CAD build for the part. Positions are in the model's coordinates, mm. Face numbers are marked on the shaded views. A direction names the side the tool comes from. Round coordinates to 2 decimals unless told otherwise and drop trailing zeros. Loops run counter-clockwise (first coordinate to the right, second up) from the corner with the lowest first, then second, coordinate; pieces in that order, holes last. Notation, with made-up numbers: (83.25, 23) -> (108.25, 23) arc R34 ccw to (108.25, 61) -> close; hole circle Ø5 at (6, 24.5). An arc over 180 degrees is marked (long way). Answer as CSV lines item,"result".
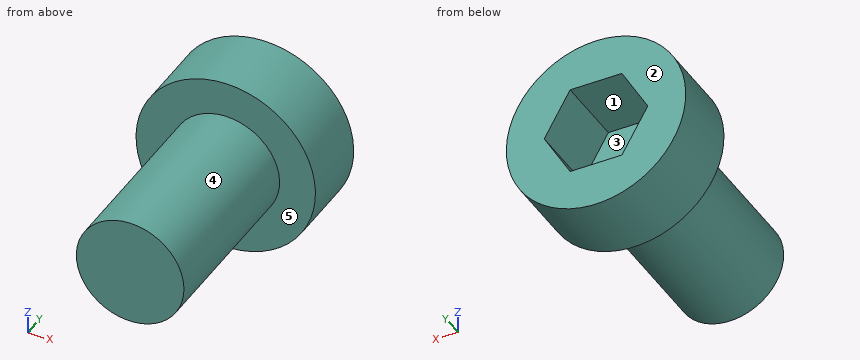
```python
from build123d import *

# Parameters (mm, degrees)
SKETCH1_R      = 3
EXTRUDE1_DEPTH = 10
SKETCH2_R      = 5
EXTRUDE2_DEPTH = 4


with BuildPart() as part:
    # Sketch1 → Extrude1 (new body)
    with BuildSketch(Plane(origin=(0, 0, 0), x_dir=(1, 0, 0), z_dir=(0, 1, 0))):
        with Locations(Location((0, 0, 0), (0, 0, 270))):
            Circle(SKETCH1_R)
    extrude(amount=-EXTRUDE1_DEPTH)

    # Sketch2 → Extrude2 (add)
    with BuildSketch(Plane(origin=(0, 0, 0), x_dir=(1, 0, 0), z_dir=(0, 1, 0))):
        with Locations(Location((0, 0, 0), (0, 0, 270))):
            Circle(SKETCH2_R)
        Polygon((2.886751346, 0), (1.443375673, 2.5), (-1.443375673, 2.5), (-2.886751346, 0), (-1.443375673, -2.5), (1.443375673, -2.5), align=None, mode=Mode.SUBTRACT)
    extrude(amount=EXTRUDE2_DEPTH)


solid = part.part
```
Q1. Slice it at D-D, the plane y = -4.5. Give the cut face in (x, z).
Results:
outline,"circle Ø6 at (0, 0)"
Q2. Slice it at B-B, the plane x = 0. Give the cut face in (y, z).
Results:
outline,"(-10, -3) -> (0, -3) -> (0, -5) -> (4, -5) -> (4, -2.5) -> (0, -2.5) -> (0, 2.5) -> (4, 2.5) -> (4, 5) -> (0, 5) -> (0, 3) -> (-10, 3) -> close"
Q3. Probe L1, parallel to Y at x = 0.75, z = 0; L2, parallel to Y at x = 2.75, z = -2; L3, parallel to Z at x = 2.75, y = 3.25. List the from-to ranges inside material, lowest first. Write a range as [from, to].
Results:
L1,"[-10, 0]"
L2,"[0, 4]"
L3,"[-4.18, -0.24], [0.24, 4.18]"
Q4. Two-plate mould, pull along X, no slides. Class the marked faces 3, 4 and 5: pulls with the +X half, pulls with the -X half, needs draft (parallel to the pull), parting line crosses it, or undercut.
Results:
face 3,"undercut"
face 4,"parting line crosses it"
face 5,"needs draft"
Q5. Drop flat-ended pins along their axis: pin 1 Ø4 at (x, y) = (1.5, -7.5) entering from -Z; pin 2 Ø1.5 at (x, z) = (0.5, -0.5) entering from +Y; pin 3 Ø2 at (y, z) = (-6.5, -3.5) entering from -X. Give the stop position or say it passes through.
Results:
pin 1,"z = -3"
pin 2,"y = 0"
pin 3,"x = -1.66"
Q6. Slice it at C-C, the plane z = 0.25. Give the cut face in (x, y), and give its area (3 significant figures).
Results:
outline,"(-4.99, 0) -> (-2.99, 0) -> (-2.99, -10) -> (2.99, -10) -> (2.99, 0) -> (4.99, 0) -> (4.99, 4) -> (2.74, 4) -> (2.74, 0) -> (-2.74, 0) -> (-2.74, 4) -> (-4.99, 4) -> close"
area,"77.8 mm2"
Q7. Tool access for the marked faces 1 and 2: list every direction of +Z, -Z, +X, -X, +Y, -Y with a clear straight run to the whole face (end or side of a thin tool).
Results:
face 1,"+Y"
face 2,"+Z, -Z, +X, -X, +Y"
Q8. Slice it at A-A, the plane y = 2. Give the cut face in (x, z).
Results:
outline,"circle Ø10 at (0, 0); hole (-2.89, 0) -> (-1.44, -2.5) -> (1.44, -2.5) -> (2.89, 0) -> (1.44, 2.5) -> (-1.44, 2.5) -> close"
